Answer from the drawing. Dimensions are ordinates in mm from the lowest x, y and z of the part. Give positions to 0.01 mm unless a question says otherwise; leave off trailing zeros. Loops run counter-clockwise (first coordinate to the right, second up) from the corner with the lowest first, then second, coordinate; pieces in that order, holes last. Notation, with made-up numbers: M 3,3 L 12,3 A27 ccw 12,27 Z; hole C 20.5,46.5 d9. An arc over 180 degrees is marked long. Use a Markdown table: item, result.
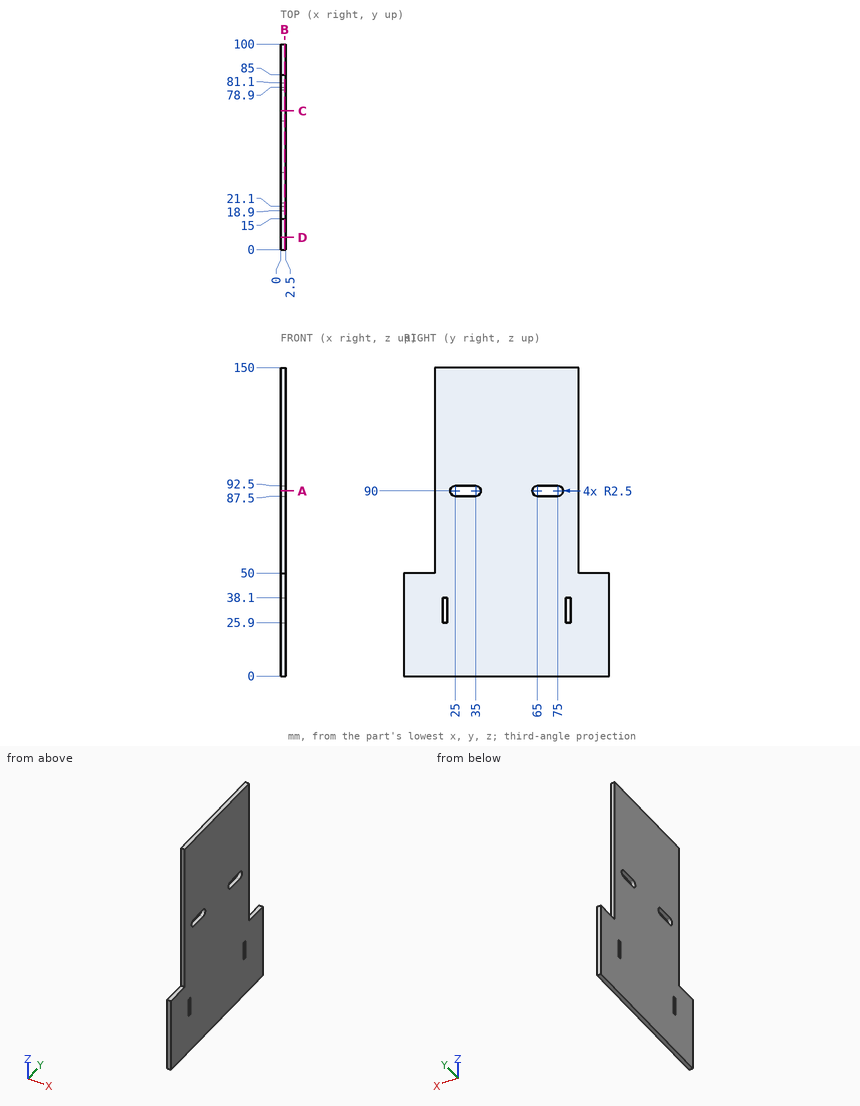
(1) A cutting plane is placed at A-A (z = 90). Write down the section's boundary in (x, y), and give its area (3 significant figures).
Entries:
| item | result |
|---|---|
| outline | M 0,15 L 2.5,15 L 2.5,22.5 L 0,22.5 Z; M 0,37.5 L 2.5,37.5 L 2.5,62.5 L 0,62.5 Z; M 0,77.5 L 2.5,77.5 L 2.5,85 L 0,85 Z |
| area | 100 mm² |
(2) Consider probe 1 along Y at (x, z) = (2.1, 32); probe 2 along Z at (x, y) = (1, 68); probe 3 along Z at (x, y) = (1.8, 81). Determine where each line is inside the solid, lowest interval first. Write a range as [from, to].
Entries:
| item | result |
|---|---|
| probe 1 | y = [0, 18.9], [21.1, 78.9], [81.1, 100] |
| probe 2 | z = [0, 87.5], [92.5, 150] |
| probe 3 | z = [0, 25.9], [38.1, 150] |
(3) Given P1, Ø1.2, axis at x = 1.5, z = 108, coming from the -Y side; P2, Ø0.8, axis at x = 1.5, y = 94.5, coming from the +Z side, each flat-ended and moving along its own axis, determine where each tip first touches the part or whether it passes through.
Entries:
| item | result |
|---|---|
| P1 | stops at y = 15 |
| P2 | stops at z = 50 |
(4) A cutting plane is placed at C-C (y = 67.5). Write down the section's boundary in (x, z).
Entries:
| item | result |
|---|---|
| outline | M 0,0 L 2.5,0 L 2.5,87.5 L 0,87.5 Z; M 0,92.5 L 2.5,92.5 L 2.5,150 L 0,150 Z |
(5) A cutting plane is placed at B-B (x = 2). Write down the section's boundary in (y, z), and give its area (3 significant figures).
Entries:
| item | result |
|---|---|
| outline | M 0,0 L 100,0 L 100,50 L 85,50 L 85,150 L 15,150 L 15,50 L 0,50 Z; hole M 18.9,25.9 L 21.1,25.9 L 21.1,38.1 L 18.9,38.1 Z; hole M 25,87.5 L 35,87.5 A2.5 ccw 35,92.5 L 25,92.5 A2.5 ccw Z; hole M 65,87.5 L 75,87.5 A2.5 ccw 75,92.5 L 65,92.5 A2.5 ccw Z; hole M 78.9,25.9 L 81.1,25.9 L 81.1,38.1 L 78.9,38.1 Z |
| area | 11,800 mm² |
(6) A cutting plane is placed at D-D (y = 6). Write down the section's boundary in (x, z).
Entries:
| item | result |
|---|---|
| outline | M 0,0 L 2.5,0 L 2.5,50 L 0,50 Z |
